Could you check a few things on this model? Use its own coordinates, in mm. A direction names the side the tool comes from. Give positions to 0.01 mm unless a question says otherwise; leave off trailing zeros. Order: outer loops, then holes, each group sorted by start corner. A loop starts at its lowest first (then second) coordinate and runs counter-clockwise, first axis right, second up.
(1) Imagine slicing it at D-D, the plane x = 7.5. Write out the boundary of the cut face in (y, z).
(2) Imagine slicing it at A-A, the plane x = 25.4. Write out the boundary of the cut face in (y, z), then the cut area to 3 significant figures.
(3) On a 3-axis mill with a long thin cutter (end or side, diameter ignored), from which of +Z, -Z, +X, -X, +Y, -Y can I reach the whole of each face in a straight line? I mean faces 4 (the flat face through (12.7, -10, 22)), 5 (the flat face through (38.1, -10, 22)), 6 (the flat face through (0, -13, 3)). Say none if no direction works.
(4) Imagine slicing it at B-B, the plane z = 21. Write out the boundary of the cut face in (x, y), then the cut area to 3 significant figures.
(5) If we mould it in two halves opening along Y, with no side actions, what happens to faces 1 (the flat face through (25, -19.05, 19)), 2 (the flat face through (25, -20, 6.35)), 3 (the cylindrical face through (7.679, -22.113, 3.219))? For each: released by +Y, released by -Y, zero draft, split by the parting line, or undercut.
(6) If I drill on probe 1 along Z at (x, y) = (25, -7); probe 2 along X at (y, z) = (-24.5, 2.5); probe 3 along Z at (x, y) = (41, -23.5), over which ranges is the centre line in solid material (lowest first)?
(7) Will these pins go through, and if not, where does the flat tip stop? pin 1 (9.5 mm diameter, centred on y = -9, z = 25, fed in from +X); pin 2 (11.5 mm diameter, centred on x = 25.4, z = 26.38, fed in from +Y); pin 3 (12 mm diameter, centred on y = -22.5, z = 15, fed in from -X); pin 4 (9.5 mm diameter, centred on y = -13, z = 22, fed in from -X).
from build123d import *

# Parameters (mm, degrees)
F0_W      = 50.8
F0_H      = 44.45
F1_DEPTH  = 31.75
F2_W      = 50.8
F2_H      = 12.7
F3_DEPTH  = 38.1
F5_DEPTH  = 25.4
F7_DEPTH  = 25.4
F8_R      = 6.35
F9_DEPTH  = 25.4
F11_DEPTH = 25.4
F12_R     = 1.8359706644
F12_R_2   = 1.6334944076
F13_DEPTH = 25.4


with BuildPart() as f1:
    # F0 (on Front) → F1 (new body)
    with BuildSketch(Plane.XZ):
        with Locations((25.4, 22.225)):
            Rectangle(F0_W, F0_H)
    extrude(amount=F1_DEPTH)

    # F2 (on face) → F3 (cut)
    with BuildSketch(Plane.XY.offset(44.45)):
        with Locations((25.4, -25.4)):
            Rectangle(F2_W, F2_H)
    extrude(amount=-F3_DEPTH, mode=Mode.SUBTRACT)

    # F4 (on face) → F5 (cut)
    with BuildSketch(Plane.XZ.offset(19.05)):
        with BuildLine():
            Line((12.7, 12.7), (12.7, 44.45))
            Line((12.7, 44.45), (0, 44.45))
            Line((0, 44.45), (0, 6.35))
            Line((0, 6.35), (9.525, 6.35))
            ThreePointArc((9.525, 6.35), (11.8620158286, 9.1502420857), (12.7, 12.7))
        make_face()
        with BuildLine():
            Line((50.8, 44.45), (38.1, 44.45))
            Line((38.1, 44.45), (38.1, 12.7))
            ThreePointArc((38.1, 12.7), (38.9379841714, 9.1502420857), (41.275, 6.35))
            Line((41.275, 6.35), (50.8, 6.35))
            Line((50.8, 6.35), (50.8, 44.45))
        make_face()
    extrude(amount=-F5_DEPTH, mode=Mode.SUBTRACT)

    # F6 (on face) → F7 (cut)
    with BuildSketch(Plane.XZ.offset(19.05)):
        with BuildLine():
            ThreePointArc((12.7, 31.75), (25.4, 39.0829550295), (38.1, 31.75))
            Line((38.1, 31.75), (38.1, 44.45))
            Line((38.1, 44.45), (12.7, 44.45))
            Line((12.7, 44.45), (12.7, 31.75))
        make_face()
    extrude(amount=-F7_DEPTH, mode=Mode.SUBTRACT)

    # F8 (on face) → F9 (cut)
    with BuildSketch(Plane.XZ.offset(19.05)):
        with Locations((25.4, 26.3829550295)):
            Circle(F8_R)
    extrude(amount=-F9_DEPTH, mode=Mode.SUBTRACT)

    # F10 (on face) → F11 (cut)
    with BuildSketch(Plane.XY.offset(6.35)):
        with BuildLine():
            ThreePointArc((6.9156312384, -31.75), (2.4537189806, -29.7044848728), (0, -25.4533607513))
            Line((0, -25.4533607513), (0, -31.75))
            Line((0, -31.75), (6.9156312384, -31.75))
        make_face()
        with BuildLine():
            ThreePointArc((50.8, -26.9937257878), (49.186939224, -30.097358798), (46.1042001843, -31.75))
            Line((46.1042001843, -31.75), (50.8, -31.75))
            Line((50.8, -31.75), (50.8, -26.9937257878))
        make_face()
    extrude(amount=-F11_DEPTH, mode=Mode.SUBTRACT)

    # F12 (on face) → F13 (cut)
    with BuildSketch(Plane.XY.offset(6.35)):
        with Locations((44.9713739546, -25.9353929963)):
            Circle(F12_R)
        with Locations((7.8915055924, -23.7321358982)):
            Circle(F12_R_2)
    extrude(amount=-F13_DEPTH, mode=Mode.SUBTRACT)


solid = f1.part
Answer block:
1. outline: (-31.75, 0) - (-25.32, 0) - (-25.32, 6.35) - (-31.75, 6.35) - close; (-22.15, 0) - (0, 0) - (0, 6.35) - (-22.15, 6.35) - close
2. outline: (-31.75, 0) - (0, 0) - (0, 20.03) - (-19.05, 20.03) - (-19.05, 6.35) - (-31.75, 6.35) - close; (-19.05, 32.73) - (0, 32.73) - (0, 39.08) - (-19.05, 39.08) - close
2. area: 583 mm2
3. face 4: +Z, -X, +Y, -Y
3. face 5: +Z, +X, +Y, -Y
3. face 6: +Z, -Z, -X, +Y, -Y
4. outline: (12.7, -19.05) - (22.03, -19.05) - (22.03, 0) - (12.7, 0) - close; (28.77, -19.05) - (38.1, -19.05) - (38.1, 0) - (28.77, 0) - close
4. area: 356 mm2
5. face 1: released by -Y
5. face 2: zero draft
5. face 3: undercut
6. probe 1: z = 0 to 20.05, 32.72 to 39.08
6. probe 2: x = 0 to 6.45, 9.33 to 43.83, 46.12 to 50.8
6. probe 3: z = 0 to 6.35
7. pin 1: stops at x = 38.1
7. pin 2: passes through
7. pin 3: stops at x = 12.26
7. pin 4: stops at x = 12.7
